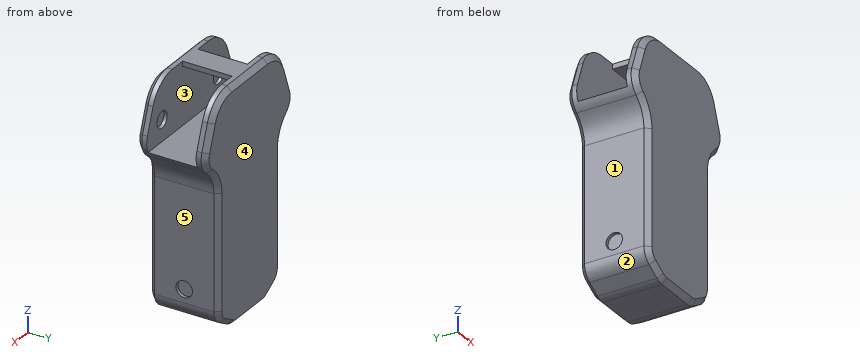
from build123d import *

# Parameters (mm, degrees)
BOSS_EXTRUDE1_DEPTH      = 21
BOSS_EXTRUDE1_DEPTH_BACK = 21
CUT_EXTRUDE2_DEPTH       = 150.699259177
CUT_EXTRUDE2_DEPTH_BACK  = 150.699259177
SKETCH3_W                = 38
SKETCH3_H                = 30
CHAMFER1_SIZE            = 3
BOSS_EXTRUDE2_REACH      = 154.528
SKETCH4_W                = 15
SKETCH4_H                = 3
SKETCH5_R                = 5
CUT_EXTRUDE3_DEPTH       = 2
SKETCH6_R                = 5
CUT_EXTRUDE4_DEPTH       = 2


with BuildPart() as part:
    # Sketch1 → Boss-Extrude1 (new, two sides: drawn at the far end of the back side and taken through both)
    with BuildSketch(Plane(origin=(0, 0, 0), x_dir=(1, 0, 0), z_dir=(0, 1, 0)).offset(-BOSS_EXTRUDE1_DEPTH_BACK)):
        with BuildLine():
            Line((12.320508076, 0), (-12.320508076, 0))
            ThreePointArc((-12.320508076, 0), (-14.908698527, -0.340741737), (-17.320508076, -1.339745962))
            Line((-17.320508076, -1.339745962), (-25, -5.773502692))
            ThreePointArc((-25, -5.773502692), (-28.660254038, -9.43375673), (-30, -14.43375673))
            Line((-30, -14.43375673), (-30, -84.024253192))
            ThreePointArc((-30, -84.024253192), (-32.022876143, -92.789127283), (-37.682301783, -99.780975904))
            ThreePointArc((-37.682301783, -99.780975904), (-42, -106.185164374), (-41.729898157, -113.904179391))
            Line((-41.729898157, -113.904179391), (-36.257575864, -128.939261324))
            ThreePointArc((-36.257575864, -128.939261324), (-28.928358883, -138.413184128), (-17.5, -142))
            Line((-17.5, -142), (17.5, -142))
            ThreePointArc((17.5, -142), (28.928358883, -138.413184128), (36.257575864, -128.939261324))
            Line((36.257575864, -128.939261324), (41.729898157, -113.904179391))
            ThreePointArc((41.729898157, -113.904179391), (42, -106.185164374), (37.682301783, -99.780975904))
            ThreePointArc((37.682301783, -99.780975904), (32.022876143, -92.789127283), (30, -84.024253192))
            Line((30, -84.024253192), (30, -14.43375673))
            ThreePointArc((30, -14.43375673), (28.660254038, -9.43375673), (25, -5.773502692))
            Line((25, -5.773502692), (17.320508076, -1.339745962))
            ThreePointArc((17.320508076, -1.339745962), (14.908698527, -0.340741737), (12.320508076, 0))
        make_face()
    extrude(amount=BOSS_EXTRUDE1_DEPTH + BOSS_EXTRUDE1_DEPTH_BACK)

    # Sketch3 → Cut-Extrude2 (cut, two sides: drawn at the far end of the back side and taken through both)
    with BuildSketch(Plane(origin=(0, 0, 0), x_dir=(0, 0, -1), z_dir=(1, 0, 0)).offset(-CUT_EXTRUDE2_DEPTH_BACK)):
        with Locations((-123, 0)):
            Rectangle(SKETCH3_W, SKETCH3_H)
    extrude(amount=CUT_EXTRUDE2_DEPTH + CUT_EXTRUDE2_DEPTH_BACK, mode=Mode.SUBTRACT)

    # Chamfer1
    chamfer1_edges = [part.edges().sort_by_distance(p)[0] for p in [
        (-38.99373701, -21, 121.421720357),
        (-28.928358883, -21, 138.413184128),
        (0, -21, 142),
        (28.928358883, -21, 138.413184128),
        (38.99373701, -21, 121.421720357),
        (42, -21, 106.185164374),
        (32.022876143, -21, 92.789127283),
        (30, -21, 49.229004961),
        (28.660254038, -21, 9.43375673),
        (21.160254038, -21, 3.556624327),
        (-32.022876143, -21, 92.789127283),
        (-32.022876143, 21, 92.789127283),
        (-42, 21, 106.185164374),
        (-38.99373701, 21, 121.421720357),
        (-28.928358883, 21, 138.413184128),
        (0, 21, 142),
        (28.928358883, 21, 138.413184128),
        (38.99373701, 21, 121.421720357),
        (42, 21, 106.185164374),
        (14.908698527, -21, 0.340741737),
        (32.022876143, 21, 92.789127283),
        (30, 21, 49.229004961),
        (28.660254038, 21, 9.43375673),
        (21.160254038, 21, 3.556624327),
        (14.908698527, 21, 0.340741737),
        (0, 21, 0),
        (-14.908698527, 21, 0.340741737),
        (-21.160254038, 21, 3.556624327),
        (-28.660254038, 21, 9.43375673),
        (-30, 21, 49.229004961),
        (0, -21, 0),
        (-14.908698527, -21, 0.340741737),
        (-21.160254038, -21, 3.556624327),
        (-28.660254038, -21, 9.43375673),
        (-30, -21, 49.229004961),
        (-42, -21, 106.185164374),
    ]]
    chamfer(chamfer1_edges, length=CHAMFER1_SIZE)

    # Sketch4 → Boss-Extrude2 (add, up to next)
    with BuildSketch(Plane(origin=(0, -15, 0), x_dir=(1, 0, 0), z_dir=(0, 1, 0)), mode=Mode.PRIVATE) as boss_extrude2_sk1:
        with Locations((0, -140.5)):
            Rectangle(SKETCH4_W, SKETCH4_H)
    boss_extrude2_tool1 = extrude(boss_extrude2_sk1.sketch, amount=BOSS_EXTRUDE2_REACH, mode=Mode.PRIVATE) - part.part
    add(boss_extrude2_tool1.solids().sort_by_distance((0, -15, 140.5))[0])

    # Sketch5 → Cut-Extrude3 (cut)
    with BuildSketch(Plane(origin=(0, -15, 0), x_dir=(1, 0, 0), z_dir=(0, 1, 0))):
        with Locations(Location((-27.5, -117, 0), (0, 0, 270))):
            Circle(SKETCH5_R)
        with Locations(Location((27.5, -117, 0), (0, 0, 90))):
            Circle(SKETCH5_R)
    extrude(amount=-CUT_EXTRUDE3_DEPTH, mode=Mode.SUBTRACT)

    # Sketch6 → Cut-Extrude4 (cut)
    with BuildSketch(Plane.ZY.offset(30)):
        with Locations((22.5, 0)):
            Circle(SKETCH6_R)
    cut_extrude4 = extrude(amount=-CUT_EXTRUDE4_DEPTH, mode=Mode.SUBTRACT)

    # Mirror1: Cut-Extrude4 across plane
    add(cut_extrude4.mirror(Plane(origin=(0, 0, 0), x_dir=(0, 0, 1), z_dir=(1, 0, 0))), mode=Mode.SUBTRACT)


solid = part.part
Can you work these out from the model? Positions are in its coordinate system, mm. Face numbers are marked on the shaded views. A direction names the side the tool comes from. Coordinates: 2 decimals unless noted, no trailing zeros. Loops run counter-clockwise (first coordinate to the right, second up) from the corner with the lowest first, then second, coordinate; pieces in that order, holes last. Notation, with made-up numbers: (-22.5, 6.25) - (-18.5, 6.25) arc R31 ccw to (-18.5, 45.25) - close; hole circle Ø5 at (28.25, 19.25). An arc over 180 degrees is marked (long way). Answer as a JSON object with one key per item and string values. Group by question number.
Item 1: If I drill on L1, parallel to Z at x = 7, y = -1; L2, parallel to Y at x = 5, z = 113; L3, parallel to X at y = -15.5, z = 117, over which ranges is the centre line in solid material (lowest first)? Write a range as from..to.
Item 2: If we section it at B-B (x = 2): List the corners of the cut face in (y, z) for me.
Item 3: If we section it at D-D (z = 117): List the corners of the cut face in (x, y) for me.
Item 4: On a 3-axis mill with a long thin cutter (end or side, diameter ignored), from which of +Z, -Z, +X, -X, +Y, -Y can I reach the whole of each face in a straight line? I mean the marked faces 4 and 5. Say none if no direction works.
Item 5: If we section it at A-A (y = 0): List the corners of the cut face in (x, z) for me, plus the area to 3 significant figures.
Item 6: If we section it at C-C (z = 22.5): List the corners of the cut face in (x, y) for me, plus the area to 3 significant figures.
Item 7: For pin 1 (5 mm diameter, centred on x = -15, y = 1.5, fed in from +Z); pin 2 (12 mm diameter, centred on y = -11, z = 91, fed in from -X); pin 3 (4 mm diameter, centred on x = -24, y = 7.5, fed in from -Z), each with a flat end and sliding along its axis, tell me the tip position at first contact or that it passes through.
Item 8: If we mould it in two halves opening along Z, with no side actions, what happens to the marked faces 1, 2 and 3? For each: released by +Z, released by -Z, zero draft, split by the parting line, or undercut.
Returned:
{
 "1": {"L1": "z = 0..104, 139..142", "L2": "y = -21..-15, 15..21", "L3": "x = -40.6..-32.5, -22.5..22.5, 32.5..40.6"},
 "2": {"outline": "(-21, 3) - (-18, 0) - (18, 0) - (21, 3) - (21, 139) - (18, 142) - (-18, 142) - (-21, 139) - close; hole (-15, 104) - (15, 104) - (15, 139) - (-15, 139) - close"},
 "3": {"outline": "(-40.6, -18) - (-37.41, -21) - (37.41, -21) - (40.6, -18) - (40.6, -15) - (32.5, -15) - (32.5, -17) - (22.5, -17) - (22.5, -15) - (-22.5, -15) - (-22.5, -17) - (-32.5, -17) - (-32.5, -15) - (-40.6, -15) - close; (-40.6, 15) - (40.6, 15) - (40.6, 18) - (37.41, 21) - (-37.41, 21) - (-40.6, 18) - close"},
 "4": {"face 4": "+Z, -Z, +X, -X, +Y", "face 5": "-Z, +X, +Y, -Y"},
 "5": {"outline": "(-41.14, 104) arc R12.5 ccw to (-37.68, 99.78) arc R20 cw to (-30, 84.02) - (-30, 27.5) - (-28, 27.5) - (-28, 17.5) - (-30, 17.5) - (-30, 14.43) arc R10 ccw to (-25, 5.77) - (-17.32, 1.34) arc R10 ccw to (-12.32, 0) - (12.32, 0) arc R10 ccw to (17.32, 1.34) - (25, 5.77) arc R10 ccw to (30, 14.43) - (30, 17.5) - (28, 17.5) - (28, 27.5) - (30, 27.5) - (30, 84.02) arc R20 cw to (37.68, 99.78) arc R12.5 ccw to (41.14, 104) - close; (-7.5, 139) - (7.5, 139) - (7.5, 142) - (-7.5, 142) - close", "area": "6,260 mm²"},
 "6": {"outline": "(-30, -18) - (-27, -21) - (27, -21) - (30, -18) - (30, -5) - (28, -5) - (28, 5) - (30, 5) - (30, 18) - (27, 21) - (-27, 21) - (-30, 18) - (-30, 5) - (-28, 5) - (-28, -5) - (-30, -5) - close", "area": "2,460 mm²"},
 "7": {"pin 1": "stops at z = 104", "pin 2": "stops at x = -34.78", "pin 3": "stops at z = 4.04"},
 "8": {"face 1": "zero draft", "face 2": "released by -Z", "face 3": "undercut"}
}
